For this review, use the dimensioned drawing (mm, ordinates from the lowest corner) and the shaded views. A direction names the side the tool comes from. Give positions to 0.01 mm unless a question says otherwise; leave off trailing zeros. Loops run counter-clockwise (first coordinate to the right, second up) from the corner with the lowest first, then second, coordinate; pieces in that order, holes last. Notation, with made-up numbers: (69, 64) - (106, 64) arc R28 ccw to (106, 89) - close; hole circle Ø1 at (3.25, 5). An arc over 180 degrees is marked (long way). Put each result on its own line as item: value.
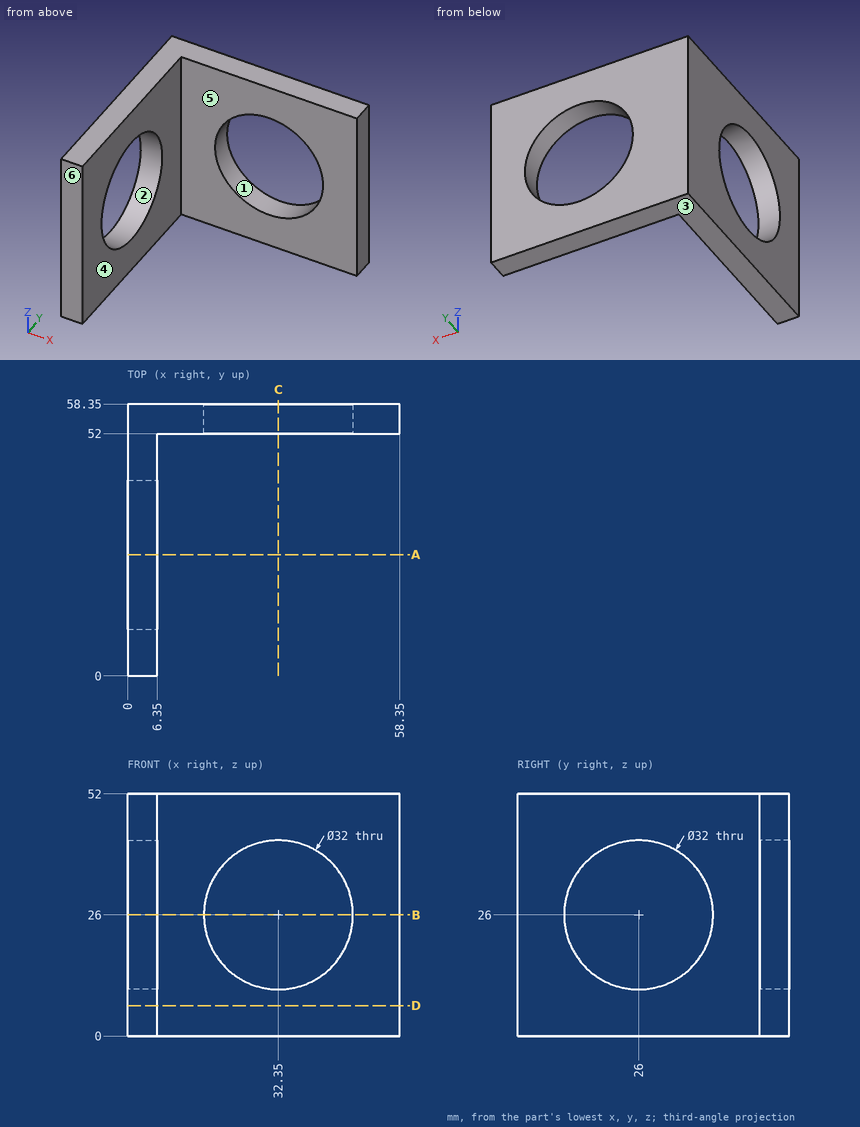
1) Take a section at D-D on z = 6.5. State the section outline as (x, y) points, and give its area (3 significant figures).
Geometry check:
outline: (0, 0) - (6.35, 0) - (6.35, 52) - (58.35, 52) - (58.35, 58.35) - (0, 58.35) - close
area: 701 mm²
2) For the marked faces 5 and 6, list the 3-axis set-ups (+Z, -Z, +X, -X, +Y, -Y) from which the entire face can be reached by the end or side of a thin tool; tool diameter is ignored.
Geometry check:
face 5: +Z, -Z, +X, -Y
face 6: +Z, -Z, +X, -X, -Y
3) Take a section at B-B on z = 26. State the section outline as (x, y) points.
Geometry check:
outline: (0, 0) - (6.35, 0) - (6.35, 10) - (0, 10) - close; (0, 42) - (6.35, 42) - (6.35, 52) - (16.35, 52) - (16.35, 58.35) - (0, 58.35) - close; (48.35, 52) - (58.35, 52) - (58.35, 58.35) - (48.35, 58.35) - close
4) Draft analysis for pull direction Z (two halves, no side actions). For the marked faces 1, 2, 3 and 4, state which applies: pulls with the +Z half, pulls with the -Z half, needs draft (parallel to the pull), parting line crosses it, or undercut.
Geometry check:
face 1: undercut
face 2: undercut
face 3: pulls with the -Z half
face 4: needs draft
5) Take a section at C-C on x = 32.35. State the section outline as (y, z) points.
Geometry check:
outline: (52, 0) - (58.35, 0) - (58.35, 10) - (52, 10) - close; (52, 42) - (58.35, 42) - (58.35, 52) - (52, 52) - close
6) Wall thickness on line 1 (Z direction, x = 32.35, y = 55); line 2 (X direction, y = 53.5, z = 26); line 3 (Y direction, x = 4, z = 26): over which ranges is each line inside the solid? List them lowest first.
Geometry check:
line 1: z = 0 to 10, 42 to 52
line 2: x = 0 to 16.35, 48.35 to 58.35
line 3: y = 0 to 10, 42 to 58.35
7) Take a section at A-A on y = 26. State the section outline as (x, z) points.
Geometry check:
outline: (0, 0) - (6.35, 0) - (6.35, 10) - (0, 10) - close; (0, 42) - (6.35, 42) - (6.35, 52) - (0, 52) - close
8) Insertion check: pin 1 Ø8 at (y, z) = (40.5, 16.5) entering from +X. The pin has a flat end and moves straight along its axis. Give the tip position at first contact, or say it passes through.
Geometry check:
pin 1: stops at x = 6.35
